Read the model definition and answer for the solid it produces. Units are mm, in the model's axes. Coordinates: 2 decimals unless noted, no trailing zeros. Loops run counter-clockwise (first coordinate to the right, second up) from the corner with the lowest first, then second, coordinate; pieces in that order, holes last. Notation, with made-up numbers: M 47,13 L 66,13 A15 cw 66,23 Z; hole C 88,18 d8. An arc over 180 degrees is marked long. Put each result on its own line as item: value.
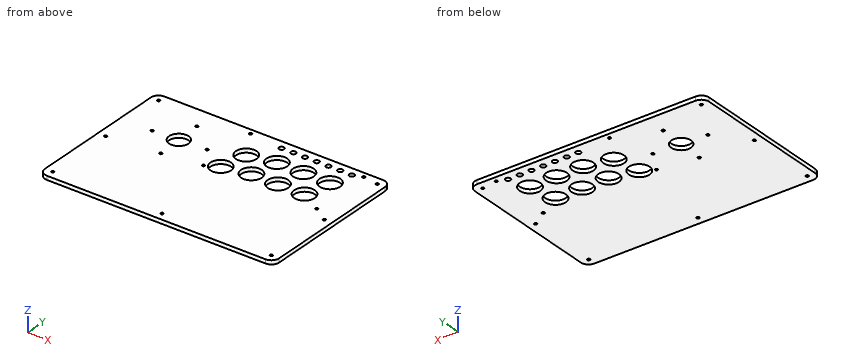
Autodesk Fusion 360 part; units mm, degrees
sketch "Sketch1" plane through (0, 0, 0) normal (0, 0, 1) x (1, 0, 0)
  line L0 (140, 100) -> (-140, 100)
  line L1 (-150, 90) -> (-150, -90)
  line L2 (-140, -100) -> (140, -100)
  line L3 (150, -90) -> (150, 90)
  line L4 (150, 100) -> (-150, -100) construction
  line L5 (-150, 100) -> (150, -100) construction
  arc A0 (-140, 100) -> (-150, 90) centre (-140, 90) ccw
  arc A1 (150, 90) -> (140, 100) centre (140, 90) ccw
  arc A2 (-150, -90) -> (-140, -100) centre (-140, -90) ccw
  arc A3 (140, -100) -> (150, -90) centre (140, -90) ccw
  circle A4 centre (-140, 90) radius 1.75
  circle A5 centre (-140, -90) radius 1.75
  circle A6 centre (140, -90) radius 1.75
  circle A7 centre (140, 90) radius 1.75
  circle A8 centre (-24.5, 93) radius 1.75
  circle A9 centre (120.5, 93) radius 1.75
  circle A10 centre (120.5, 13) radius 1.75
  circle A11 centre (-24.5, 13) radius 1.75
  circle A12 centre (-9.217, 22.009) radius 13.25
  circle A13 centre (-2.217, 56.009) radius 13.25
  circle A14 centre (24.783, 29.009) radius 13.25
  circle A15 centre (31.783, 63.009) radius 13.25
  circle A16 centre (65.783, 63.009) radius 13.25
  circle A17 centre (58.783, 29.009) radius 13.25
  circle A18 centre (92.783, 29.009) radius 13.25
  circle A19 centre (99.783, 63.009) radius 13.25
  circle A20 centre (108.5, 88.75) radius 3.25
  circle A21 centre (93.5, 88.75) radius 3.25
  circle A22 centre (78.5, 88.75) radius 3.25
  circle A23 centre (63.5, 88.75) radius 3.25
  circle A24 centre (33.5, 88.75) radius 3.25
  circle A25 centre (48.5, 88.75) radius 3.25
  circle A26 centre (18.5, 88.75) radius 3.25
  circle A27 centre (-75.717, 39.009) radius 12.5
  circle A28 centre (-77.417, 71.909) radius 1.75
  circle A29 centre (-108.617, 37.309) radius 1.75
  circle A30 centre (-74.017, 6.109) radius 1.75
  circle A31 centre (-40.817, 40.709) radius 1.75
  circle A32 centre (-140, 0) radius 1.75
  circle A33 centre (140, 0) radius 1.75
  circle A34 centre (0, -90) radius 1.75
  dimension "d1" = 300
  dimension "d2" = 200
  dimension "d3" = 10
  dimension "d4" = 10
  dimension "d5" = 10
  dimension "d6" = 10
  dimension "d7" = 3.5
  dimension "d8" = 3.5
  dimension "d9" = 3.5
  dimension "d10" = 3.5
  dimension "d13" = 3.5
  dimension "d14" = 145
  dimension "d15" = 3.5
  dimension "d16" = 3.5
  dimension "d17" = 145
  dimension "d18" = 3.5
  dimension "d21" = 26.5
  dimension "d22" = 26.5
  dimension "d23" = 26.5
  dimension "d24" = 26.5
  dimension "d25" = 26.5
  dimension "d26" = 26.5
  dimension "d27" = 26.5
  dimension "d28" = 26.5
  dimension "d31" = 6.5
  dimension "d32" = 6.5
  dimension "d33" = 6.5
  dimension "d34" = 6.5
  dimension "d35" = 6.5
  dimension "d36" = 6.5
  dimension "d37" = 6.5
  dimension "d41" = 25
  dimension "d44" = 3.5
  dimension "d58" = 3.5
  dimension "d59" = 3.5
  dimension "d60" = 3.5
sketch "Sketch2" plane through (0, 0, 5) normal (0, 0, 1) x (-1, 0, 0)
  circle A0 centre (77.417, -71.909) radius 1.75
  circle A1 centre (9.217, -22.009) radius 13.25
  circle A2 centre (-108.5, -88.75) radius 3.25
  circle A3 centre (-58.783, -29.009) radius 13.25
  circle A4 centre (-93.5, -88.75) radius 3.25
  circle A5 centre (40.817, -40.709) radius 1.75
  circle A6 centre (140, 90) radius 1.75
  circle A7 centre (24.5, -93) radius 1.75
  circle A8 centre (-63.5, -88.75) radius 3.25
  circle A9 centre (-18.5, -88.75) radius 3.25
  circle A10 centre (-99.783, -63.009) radius 13.25
  circle A11 centre (-33.5, -88.75) radius 3.25
  circle A12 centre (108.617, -37.309) radius 1.75
  circle A13 centre (-92.783, -29.009) radius 13.25
  circle A14 centre (-48.5, -88.75) radius 3.25
  circle A15 centre (-65.783, -63.009) radius 13.25
  circle A16 centre (140, -90) radius 1.75
  circle A17 centre (24.5, -13) radius 1.75
  circle A18 centre (-120.5, -13) radius 1.75
  circle A19 centre (-78.5, -88.75) radius 3.25
  circle A20 centre (-140, -90) radius 1.75
  circle A21 centre (-31.783, -63.009) radius 13.25
  circle A22 centre (-140, 90) radius 1.75
  circle A23 centre (74.017, -6.109) radius 1.75
  circle A24 centre (2.217, -56.009) radius 13.25
  circle A25 centre (75.717, -39.009) radius 12.5
  circle A26 centre (-120.5, -93) radius 1.75
  circle A27 centre (-24.783, -29.009) radius 13.25
  arc A28 (-140, 100) -> (-150, 90) centre (-140, 90) ccw
  line L0 (-150, 90) -> (-150, -90)
  arc A29 (-150, -90) -> (-140, -100) centre (-140, -90) ccw
  line L1 (-140, -100) -> (140, -100)
  arc A30 (140, -100) -> (150, -90) centre (140, -90) ccw
  line L2 (150, -90) -> (150, 90)
  arc A31 (150, 90) -> (140, 100) centre (140, 90) ccw
  line L3 (140, 100) -> (-140, 100)
  circle A32 centre (77.717, -62.659) radius 1.75
  circle A33 centre (99.367, -37.009) radius 1.75
  circle A34 centre (73.717, -15.359) radius 1.75
  circle A35 centre (52.067, -41.009) radius 1.75
  dimension "d53" = 3.5
  dimension "d55" = 360
extrude "Extrude4" add sketch "Sketch1" along normal blind 5
extrude "Extrude5" cut sketch "Sketch2" against normal blind 5 contours A32 | A33 | A34 | A35
sketch "Sketch3" plane through (0, 0, 5) normal (0, 0, 1) x (-1, 0, 0)
  circle A0 centre (99.367, -37.009) radius 1.75
  circle A1 centre (73.717, -15.359) radius 1.75
  circle A2 centre (77.717, -62.659) radius 1.75
  circle A3 centre (52.067, -41.009) radius 1.75
  circle A4 centre (140, 0) radius 1.75
  circle A5 centre (-63.5, -88.75) radius 3.25
  circle A6 centre (108.617, -37.309) radius 1.75
  circle A7 centre (-140, 0) radius 1.75
  circle A8 centre (-48.5, -88.75) radius 3.25
  circle A9 centre (-108.5, -88.75) radius 3.25
  circle A10 centre (24.5, -13) radius 1.75
  circle A11 centre (-78.5, -88.75) radius 3.25
  circle A12 centre (9.217, -22.009) radius 13.25
  circle A13 centre (-140, -90) radius 1.75
  circle A14 centre (2.217, -56.009) radius 13.25
  circle A15 centre (-120.5, -13) radius 1.75
  circle A16 centre (-120.5, -93) radius 1.75
  circle A17 centre (-31.783, -63.009) radius 13.25
  circle A18 centre (140, 90) radius 1.75
  circle A19 centre (75.717, -39.009) radius 12.5
  circle A20 centre (-18.5, -88.75) radius 3.25
  circle A21 centre (-58.783, -29.009) radius 13.25
  circle A22 centre (-65.783, -63.009) radius 13.25
  circle A23 centre (40.817, -40.709) radius 1.75
  circle A24 centre (24.5, -93) radius 1.75
  circle A25 centre (-140, 90) radius 1.75
  circle A26 centre (-99.783, -63.009) radius 13.25
  circle A27 centre (-92.783, -29.009) radius 13.25
  circle A28 centre (140, -90) radius 1.75
  circle A29 centre (77.417, -71.909) radius 1.75
  circle A30 centre (74.017, -6.109) radius 1.75
  circle A31 centre (-24.783, -29.009) radius 13.25
  circle A32 centre (0, 90) radius 1.75
  circle A33 centre (-33.5, -88.75) radius 3.25
  circle A34 centre (-93.5, -88.75) radius 3.25
  arc A35 (-140, 100) -> (-150, 90) centre (-140, 90) ccw
  line L0 (-150, 90) -> (-150, -90)
  arc A36 (-150, -90) -> (-140, -100) centre (-140, -90) ccw
  line L1 (-140, -100) -> (140, -100)
  arc A37 (140, -100) -> (150, -90) centre (140, -90) ccw
  line L2 (150, -90) -> (150, 90)
  arc A38 (150, 90) -> (140, 100) centre (140, 90) ccw
  line L3 (140, 100) -> (-140, 100)
extrude "Extrude6" add sketch "Sketch2" against normal up to surface (5 mm away) contours A32 | A33 | A34 | A35
extrude "Extrude1" [suppressed]
1) Find section A-A, the plane x = 63.5. Write down the section's boundary in (y, z), plus the area to 3 significant figures.
Answer list:
outline: M -100,0 L 16.63,0 L 16.63,5 L -100,5 Z; M 41.39,0 L 49.96,0 L 49.96,5 L 41.39,5 Z; M 76.06,0 L 85.5,0 L 85.5,5 L 76.06,5 Z; M 92,0 L 100,0 L 100,5 L 92,5 Z
area: 713 mm^2
2) Straight lines are drawn through the part: line 1 (Y direction, x = -140, z = 3.3); line 2 (Y direction, x = 29, z = 4.2); line 3 (X direction, y = 30, z = 3.25). For each, find the intervals that lie inside material, in ascending order. Write a range as [from, to].
Answer list:
line 1: y = [-100, -91.75], [-88.25, -1.75], [1.75, 88.25], [91.75, 100]
line 2: y = [-100, 16.45], [41.57, 50.05], [75.96, 100]
line 3: x = [-150, -84.38], [-67.05, -19.79], [1.35, 11.57], [38, 45.57], [72, 79.57], [106, 150]
3) Given pin 1 Ø16 at (x, y) = (92.783, 29.009) entering from -Z, flat-ended and moving along its own axis, determine where the tip first touches the part or whether it passes through.
Answer list:
pin 1: passes through
